Geometry check sheet. Reference: drawing and pictorial views, mm from the part's lowest x, y, z. Round coordinates to 2 decimals unless told otherwise and drop trailing zeros. Order: outer loops, then holes, each group sorted by start corner. A loop starts at its lowest first (then second) coordinate and runs counter-clockwise, first axis right, second up.
(1) Material ranges on line 1 along Y through (x, z) = (37.5, 1.1); line 2 along Y through (x, z) = (12.5, 3.5); line 3 along X through (y, z) = (8.75, 2.65), recorded low to high.
(2) Sectioned sample at B-B (y = 5.75). Record the boundary of the cut face in (x, z).
(3) Sectioned sample at C-C (z = 2). Record the boundary of the cut face in (x, y), plus the area to 3 significant figures.
(4) Sectioned sample at D-D (x = 22.5). Record the boundary of the cut face in (y, z), plus the area to 3 significant figures.
(5) Release check for a two-part mould opening along Y. For the marked faces 1, 2 and 3 record: +Y half, -Y half, draft (parallel to the pull), parting line (faces both ways), or undercut.
(6) Sectioned sample at A-A (x = 27). Record the boundary of the cut face in (y, z).
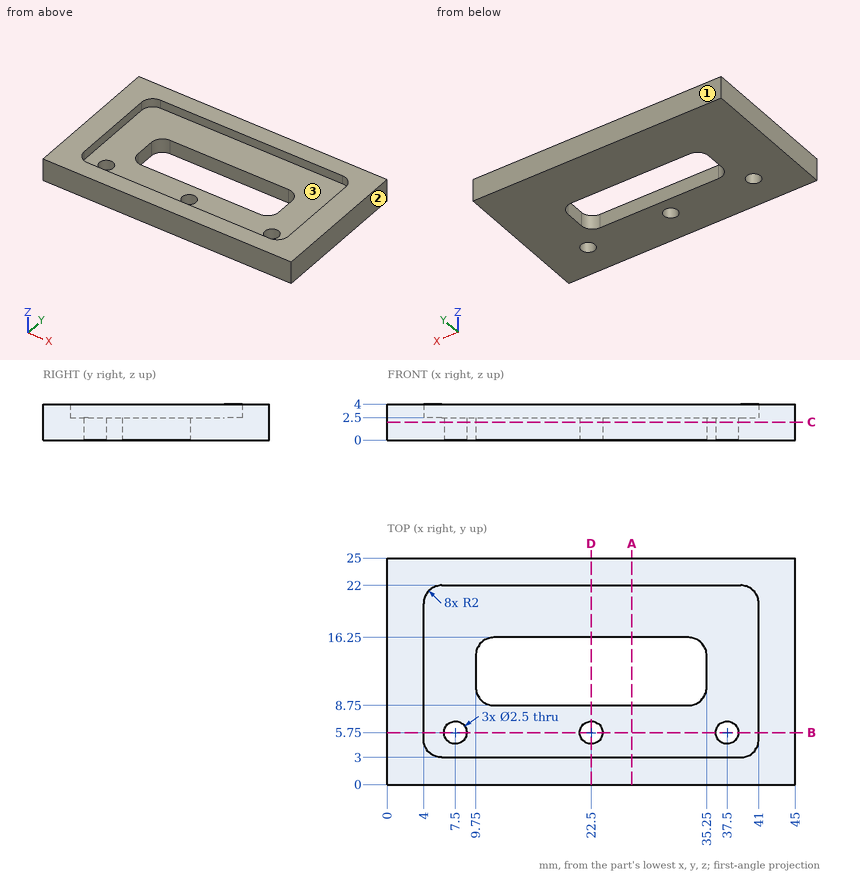
Answer below:
1. line 1: y = 0 to 4.5, 7 to 25
1. line 2: y = 0 to 3, 22 to 25
1. line 3: x = 0 to 4, 41 to 45
2. outline: (0, 0) - (6.25, 0) - (6.25, 2.5) - (4, 2.5) - (4, 4) - (0, 4) - close; (8.75, 0) - (21.25, 0) - (21.25, 2.5) - (8.75, 2.5) - close; (23.75, 0) - (36.25, 0) - (36.25, 2.5) - (23.75, 2.5) - close; (38.75, 0) - (45, 0) - (45, 4) - (41, 4) - (41, 2.5) - (38.75, 2.5) - close
3. outline: (0, 0) - (45, 0) - (45, 25) - (0, 25) - close; hole circle Ø2.5 at (7.5, 5.75); hole (9.75, 10.75) arc R2 ccw to (11.75, 8.75) - (33.25, 8.75) arc R2 ccw to (35.25, 10.75) - (35.25, 14.25) arc R2 ccw to (33.25, 16.25) - (11.75, 16.25) arc R2 ccw to (9.75, 14.25) - close; hole circle Ø2.5 at (22.5, 5.75); hole circle Ø2.5 at (37.5, 5.75)
3. area: 922 mm2
4. outline: (0, 0) - (4.5, 0) - (4.5, 2.5) - (3, 2.5) - (3, 4) - (0, 4) - close; (7, 0) - (8.75, 0) - (8.75, 2.5) - (7, 2.5) - close; (16.25, 0) - (25, 0) - (25, 4) - (22, 4) - (22, 2.5) - (16.25, 2.5) - close
4. area: 46.5 mm2
5. face 1: +Y half
5. face 2: draft
5. face 3: undercut
6. outline: (0, 0) - (8.75, 0) - (8.75, 2.5) - (3, 2.5) - (3, 4) - (0, 4) - close; (16.25, 0) - (25, 0) - (25, 4) - (22, 4) - (22, 2.5) - (16.25, 2.5) - close
